```python
from build123d import *

# Parameters (mm, degrees)
MODEL_R             = 38.5
MODEL_R_2           = 1.5
MODEL_W             = 10
MODEL_H             = 4
MODEL_W_2           = 4
MODEL_H_2           = 11.4
MODEL_W_3           = 2
MODEL_H_3           = 10
BOSS_EXTRUDE1_DEPTH = 2


with BuildPart() as part:
    # Model → Boss-Extrude1 (new body)
    with BuildSketch(Plane.XY):
        with Locations((2103.994457195, 1132.586491316)):
            Circle(MODEL_R)
        with Locations((2078.013695082, 1147.586491316)):
            Circle(MODEL_R_2, mode=Mode.SUBTRACT)
        with Locations((2129.975219309, 1147.586491316)):
            Circle(MODEL_R_2, mode=Mode.SUBTRACT)
        with Locations((2129.975219309, 1117.586491316)):
            Circle(MODEL_R_2, mode=Mode.SUBTRACT)
        with Locations((2078.013695082, 1117.586491316)):
            Circle(MODEL_R_2, mode=Mode.SUBTRACT)
        with Locations((2109.800475531, 1158.486491316)):
            Circle(MODEL_R_2, mode=Mode.SUBTRACT)
        with Locations((2109.800475531, 1110.586491316)):
            Circle(MODEL_R_2, mode=Mode.SUBTRACT)
        with Locations((2080.994457195, 1106.605729203)):
            Circle(MODEL_R_2, mode=Mode.SUBTRACT)
        with Locations((2080.994457195, 1158.56725343)):
            Circle(MODEL_R_2, mode=Mode.SUBTRACT)
        with Locations((2126.994457195, 1106.605729203)):
            Circle(MODEL_R_2, mode=Mode.SUBTRACT)
        with Locations((2126.994457195, 1158.56725343)):
            Circle(MODEL_R_2, mode=Mode.SUBTRACT)
        with Locations((2097.994457195, 1158.486491316)):
            Rectangle(MODEL_W, MODEL_H, mode=Mode.SUBTRACT)
        with Locations((2097.994457195, 1110.586491316)):
            Rectangle(MODEL_W, MODEL_H, mode=Mode.SUBTRACT)
        with Locations((2097.494457195, 1127.786491316)):
            Rectangle(MODEL_W_2, MODEL_H_2, mode=Mode.SUBTRACT)
        with Locations((2110.494457195, 1127.786491316)):
            Rectangle(MODEL_W_2, MODEL_H_2, mode=Mode.SUBTRACT)
        with BuildLine():
            Line((2101.744457195, 1132.659888489), (2101.744457195, 1122.913094144))
            ThreePointArc((2101.744457195, 1122.913094144), (2103.994457195, 1120.663094144), (2106.244457195, 1122.913094144))
            Line((2106.244457195, 1122.913094144), (2106.244457195, 1132.659888489))
            ThreePointArc((2106.244457195, 1132.659888489), (2103.994457195, 1134.909888489), (2101.744457195, 1132.659888489))
        make_face(mode=Mode.SUBTRACT)
        with Locations((2129.976886457, 1132.586491316)):
            Rectangle(MODEL_W_3, MODEL_H_3, mode=Mode.SUBTRACT)
    extrude(amount=BOSS_EXTRUDE1_DEPTH)


solid = part.part
```
Source: CAD feature listing. Evaluate the final solid. Frame: model axes, mm. Round coordinates to 2 decimals unless told otherwise and drop trailing zeros. Loops run counter-clockwise (first coordinate to the right, second up) from the corner with the lowest first, then second, coordinate; pieces in that order, holes last.
1. Section query D-D on z = 1.6. Give the number of separate pieces and of enclosed holes in the cut face, and give its area (3 significant figures).
2. Section query A-A on y = 1131. Output: boundary loops of the cut face in (x, z).
3. Mould query, pull axis Y, two halves, no side actions, for faces 1 (the flat face through (2095, 1133, 2)), 2 (the flat face through (2102.994, 1111, 1)). Classes: released by +Y, released by -Y, zero draft, split by the parting line, or undercut.
4. Section query C-C on x = 2110. Output: boundary loops of the cut face in (y, z), and give its area (3 significant figures).
5. Ray query, L1, parallel to Y at x = 2096, z = 1.2; L2, parallel to Y at x = 2110.5, z = 1.85; L3, parallel to X at y = 1111.5, z = 1.5. Return the intervals inside material, ascending.
6. Section query B-B on x = 2077.5. Output: boundary loops of the cut face in (y, z), and give its area (3 significant figures).
7. Contact query for flat-ended pins moving along their axis: pin 1 (3.5 mm diameter, centred on x = 2078.01, y = 1117.59, fed in from -Z); pin 2 (2.5 mm diameter, centred on x = 2109.8, y = 1158.49, fed in from +Z); pin 3 (1 mm diameter, centred on y = 1111.5, z = 1, fed in from -X); pin 4 (0.6 mm diameter, centred on x = 2100.5, z = 1, fed in from -Y). Output: stop coordinate, or through.
Answers below:
1. separate pieces: 1
1. enclosed holes: 16
1. area: 4,330 mm2
2. outline: (2065.53, 0) - (2095.49, 0) - (2095.49, 2) - (2065.53, 2) - close; (2099.49, 0) - (2101.74, 0) - (2101.74, 2) - (2099.49, 2) - close; (2106.24, 0) - (2108.49, 0) - (2108.49, 2) - (2106.24, 2) - close; (2112.49, 0) - (2128.98, 0) - (2128.98, 2) - (2112.49, 2) - close; (2130.98, 0) - (2142.46, 0) - (2142.46, 2) - (2130.98, 2) - close
3. face 1: zero draft
3. face 2: undercut
4. outline: (1094.56, 0) - (1109.1, 0) - (1109.1, 2) - (1094.56, 2) - close; (1112.07, 0) - (1122.09, 0) - (1122.09, 2) - (1112.07, 2) - close; (1133.49, 0) - (1157, 0) - (1157, 2) - (1133.49, 2) - close; (1159.97, 0) - (1170.62, 0) - (1170.62, 2) - (1159.97, 2) - close
4. area: 117 mm2
5. L1: y = 1094.93 to 1108.59, 1112.59 to 1122.09, 1133.49 to 1156.49, 1160.49 to 1170.25
5. L2: y = 1094.64 to 1109.26, 1111.91 to 1122.09, 1133.49 to 1157.16, 1159.81 to 1170.53
5. L3: x = 2071.78 to 2092.99, 2102.99 to 2108.61, 2110.99 to 2136.21
6. outline: (1104.65, 0) - (1116.18, 0) - (1116.18, 2) - (1104.65, 2) - close; (1119, 0) - (1146.18, 0) - (1146.18, 2) - (1119, 2) - close; (1149, 0) - (1160.52, 0) - (1160.52, 2) - (1149, 2) - close
6. area: 100 mm2
7. pin 1: stops at z = 0
7. pin 2: passes through
7. pin 3: stops at x = 2071.46
7. pin 4: stops at y = 1094.22
